Autodesk Fusion 360 part; units mm, degrees
sketch "Boceto1" plane through (0, 0, 0) normal (0, 0, 1) x (1, 0, 0)
  line L0 (2.9445, -5.1) -> (5.889, 0)
  line L1 (5.889, 0) -> (2.9445, 5.1)
  line L2 (2.9445, 5.1) -> (-2.9445, 5.1)
  line L3 (-2.9445, 5.1) -> (-5.889, 0)
  line L4 (-5.889, 0) -> (-2.9445, -5.1)
  line L5 (-2.9445, -5.1) -> (2.9445, -5.1)
  circle A0 centre (0, 0) radius 8.3
  dimension "d1" = 5.1
  dimension "d2" = 16.6
extrude "Extruir1" add sketch "Boceto1" along normal blind 8
extrude "Extruir2" add sketch "Boceto1" along normal blind 5 contours L0 L1 L2 L3 L4 L5
sketch "Boceto2" plane through (0, 0, 8) normal (0, 0, 1) x (-1, 0, 0)
  line L0 (-2.9445, 5.1) -> (2.9445, 5.1)
  line L1 (2.9445, 5.1) -> (5.889, 0)
  line L2 (5.889, 0) -> (2.9445, -5.1)
  line L3 (2.9445, -5.1) -> (-2.9445, -5.1)
  line L4 (-2.9445, -5.1) -> (-5.889, 0)
  line L5 (-5.889, 0) -> (-2.9445, 5.1)
  circle A0 centre (0, 0) radius 8.3
  circle A1 centre (0, -8.3) radius 1
  line L6 (0, 0) -> (0, -10.2342) construction
  circle A2 centre (7.188, -4.15) radius 1
  circle A3 centre (7.188, 4.15) radius 1
  circle A4 centre (0, 8.3) radius 1
  circle A5 centre (-7.188, 4.15) radius 1
  circle A6 centre (-7.188, -4.15) radius 1
  dimension "d7" = 2
  dimension "d9" = 360
extrude "Extruir3" cut sketch "Boceto2" against normal blind 8 contours A0 A3 | A0 A2 | A0 A4 | A0 A1 | A0 A5 | A0 A6 picked at (7.4639, 4.3289) picked at (7.4639, -4.3289) picked at (-0.024, 7.9631) picked at (-0.01, -8.6287) picked at (-7.4728, 4.3144) picked at (-6.9055, -3.9648)
Input: part model. Units: mm. Frame: model coordinates. A direction names the side the tool comes from. Give positions to 0.01 mm unless a question says otherwise; leave off trailing zeros. Order: outer loops, then holes, each group sorted by start corner. A loop starts at its lowest first (then second) coordinate and runs counter-clockwise, first axis right, second up. Notation, with made-up numbers: (63.25, -29) - (99.25, -29) arc R5 cw to (99.25, -23) - close; hole circle Ø9 at (-7, 71). An arc over 180 degrees is marked (long way). Answer as a JSON object with one key per item and string values. Group by question number.
Q1. Cut plane A-A, the plane z = 7.25. Output: boundary loops of the cut face in (x, y), then the cut area to 3 significant figures.
Q2. Set-up query: faces 5 (the face through (-4.396, 2.586, 6.479)), 6 (the face through (-7.3, 3.95, 3.94)). Return all of +Z, -Z, +X, -X, +Y, -Y with unobstructed straight access to the full face (end or side cutting, diameter ignored); none if empty.
Q3. Line query: probe 1 along Z at (x, y) = (0.5, 2); probe 2 along Y at (x, z) = (6.5, 0.75); probe 3 along X at (y, z) = (4.5, 6). Output: solid intervals per line, ascending.
Q4. Cut plane D-D, the plane z = 1. Output: boundary loops of the cut face in (x, y).
Q5. Cut plane B-B, the plane x = 0. Output: boundary loops of the cut face in (y, z), then the cut area to 3 significant figures.
Q6. First-contact query: pin 1 Ø3 at (x, y) = (3, 1.5) entering from +Z; pin 2 Ø1.5 at (x, z) = (0, 7) entering from -Y; pin 3 Ø1 at (y, z) = (-5, 4.5) entering from -X. Flat tips, straight axial feed; report the tip coordinate or a pass-through.
Q7. Cut plane C-C, the plane y = -4.75. Output: boundary loops of the cut face in (x, z), then the cut area to 3 significant figures.
Q8. Mould query, pull axis X, two halves, no side actions, for faces 1 (the face through (-0.1, -5.4, 8)), 2 (the face through (7.24, -4.06, 3.94)), 3 (the face through (0, 5.1, 6)), 4 (the face through (4.396, -2.586, 6.479)). Classes: pulls with the +X half, pulls with the -X half, needs draft (parallel to the pull), parting line crosses it, or undercut.
Results:
{
 "1": {"outline": "(-1, -8.24) arc R1 cw to (1, -8.24) arc R8.3 ccw to (7.63, 3.26) arc R1 cw to (6.64, 4.98) arc R8.3 ccw (long way) to start; hole (-5.89, 0) - (-2.94, -5.1) - (2.94, -5.1) - (5.89, 0) - (2.94, 5.1) - (-2.94, 5.1) - close", "area": "123 mm^2"},
 "2": {"face 5": "+Z", "face 6": "+Z, -Z"},
 "3": {"probe 1": "0 to 5", "probe 2": "-5.16 to 3.42, 4.88 to 5.16", "probe 3": "-6.97 to -3.29, 3.29 to 6.25"},
 "4": {"outline": "(-1, -8.24) arc R1 cw to (1, -8.24) arc R8.3 ccw to (7.63, 3.26) arc R1 cw to (6.64, 4.98) arc R8.3 ccw (long way) to start"},
 "5": {"outline": "(-7.3, 0) - (8.3, 0) - (8.3, 8) - (5.1, 8) - (5.1, 5) - (-5.1, 5) - (-5.1, 8) - (-7.3, 8) - close", "area": "94.2 mm^2"},
 "6": {"pin 1": "z = 5", "pin 2": "y = -7.64", "pin 3": "x = -6.97"},
 "7": {"outline": "(-6.81, 0) - (6.81, 0) - (6.81, 8) - (3.15, 8) - (3.15, 5) - (-3.15, 5) - (-3.15, 8) - (-6.81, 8) - close", "area": "90.0 mm^2"},
 "8": {"face 1": "needs draft", "face 2": "pulls with the +X half", "face 3": "undercut", "face 4": "undercut"}
}
